Can you work these out from the model? Positions are in its coordinate system, mm. Face numbers are marked on the shaded views. A direction names the side the tool comes from. Give positions to 0.01 mm unless a question says otherwise; leave off trailing zeros. Loops run counter-clockwise (first coordinate to the right, second up) from the corner with the lowest first, then second, coordinate; pieces in that order, holes last. Notation, with made-up numbers: M -3,86.25 L 44,86.25 A6 ccw 44,97.25 Z; hole C 62.25,-28.75 d1. An arc over 180 degrees is marked long. Use CSV: the item, a comma, the result in double quotes.
from build123d import *

# Parameters (mm, degrees)
PAD_DEPTH    = 11
CHAMFER_SIZE = 3
FILLET_R     = 2


with BuildPart() as part:
    # Sketch → Pad (new body)
    with BuildSketch(Plane.XY):
        Polygon((-22.800474, -3.599016), (-22.800474, -8.599016), (10.199526, -8.599016), (10.199526, 18.400984), (28.199526, 18.400984), (28.199526, -8.599016), (31.199526, -8.599016), (31.199526, 21.400984), (7.199526, 21.400984), (7.199526, -3.599016), align=None)
    extrude(amount=PAD_DEPTH)

    # Chamfer
    chamfer_edges = [part.edges().sort_by_distance(p)[0] for p in [
        (-6.300474, -8.599016, 0),
        (-6.300474, -8.599016, 11),
    ]]
    chamfer(chamfer_edges, length=CHAMFER_SIZE)

    # Fillet
    fillet_edges = [part.edges().sort_by_distance(p)[0] for p in [
        (31.199526, 21.400984, 5.5),
        (7.199526, 21.400984, 5.5),
    ]]
    fillet(fillet_edges, radius=FILLET_R)


solid = part.part
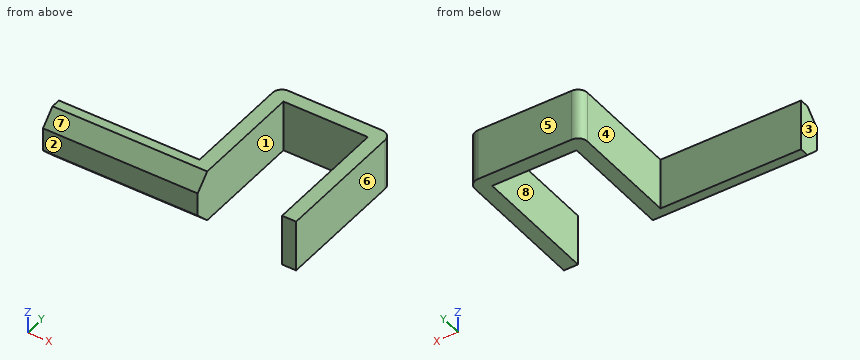
Q1. I want a section at A-A, the plane y = -4.5. Please give me the cut outline in (x, z), then the cut area to 3 significant figures.
Model answer:
outline,"M -22.8,0 L 10.2,0 L 10.2,11 L -22.8,11 Z; M 28.2,0 L 31.2,0 L 31.2,11 L 28.2,11 Z"
area,"396 mm2"
Q2. I want a section at B-B, the plane z = 4. Please give me the cut outline in (x, y), then the cut area to 3 significant figures.
Model answer:
outline,"M -22.8,-8.6 L 10.2,-8.6 L 10.2,18.4 L 28.2,18.4 L 28.2,-8.6 L 31.2,-8.6 L 31.2,19.4 A2 ccw 29.2,21.4 L 9.2,21.4 A2 ccw 7.2,19.4 L 7.2,-3.6 L -22.8,-3.6 Z"
area,"382 mm2"
Q3. If we mould it in two halves opening along X, with no side actions, what happens to the marked faces 1, 2 and 3? For each: released by +X, released by -X, zero draft, split by the parting line, or undercut.
Model answer:
face 1,"undercut"
face 2,"zero draft"
face 3,"released by -X"
Q4. I'm going to push flat-ended pins straight in: P1, Ø5.5, axis at x = 20.5, z = 8, coming from the -Y side; P2, Ø5.5, axis at y = 5.5, z = 4, coming from the -X side; P3, Ø4, axis at x = 3.5, z = 9, coming from the -Y side. Where does each tip first touch, or does it pass through?
Model answer:
P1,"y = 18.4"
P2,"x = 7.2"
P3,"y = -8.6"
Q5. For the marked faces 4, 5, 6, 7 and 8, which set-ups out of +Z, -Z, +X, -X, +Y, -Y let a thin tool reach every point of the face, with its end or its side?
Model answer:
face 4,"+Z, -Z, -X, +Y"
face 5,"+Z, -Z, +X, -X, +Y"
face 6,"+Z, -Z, +X, +Y, -Y"
face 7,"+Z, -X, -Y"
face 8,"+Z, -Z, -Y"
Q6. I want a section at C-C, the plane x = 20.5. Please give me the cut outline in (y, z).
Model answer:
outline,"M 18.4,0 L 21.4,0 L 21.4,11 L 18.4,11 Z"
Q7. Please list where these lines run through material, in increasing order: L1, parallel to X at y = 15, z = 3; L2, parallel to Y at x = 12, z = 7; L3, parallel to X at y = 18.5, z = 5. Write a range as from..to.
Model answer:
L1,"7.2..10.2, 28.2..31.2"
L2,"18.4..21.4"
L3,"7.2..31.2"
Q8. I want a section at D-D, the plane y = 1. Please give me the cut outline in (x, z).
Model answer:
outline,"M 7.2,0 L 10.2,0 L 10.2,11 L 7.2,11 Z; M 28.2,0 L 31.2,0 L 31.2,11 L 28.2,11 Z"
